The figure shows three views and two pictorial views of one solid part (mm, origin at its lowest corner). Answer the questions. Give positions to 0.01 mm unless a question says otherwise; leave off trailing zeros. Loops run counter-clockwise (first coordinate to the right, second up) from the corner with the lowest first, then second, coordinate; pieces in that order, holes last. Notation, with made-up numbers: M -28,75 L 11,75 A12 ccw 11,90 Z; hole C 86,-24.75 d6. An arc over 180 degrees is marked long. Write item = value, one per line. Start each with the question number.
1. Consider L1, parallel to Y at x = 15, z = 5.5 (3 decimals); L2, parallel to Z at x = 18.5, y = 8.75; L3, parallel to Y at x = 15, z = 17.1. Determine where each line is inside the solid, lowest interval first. Write a range as [from, to].
2. Section D-D on x = 20 is taken. Determine the outline of the cut face in (y, z), plus the area to 3 significant figures.
3. Flat-ended cylindrical pins translate along their axes: pin 1 Ø5 at (x, z) = (26, 12) entering from +Y; pin 2 Ø1 at (x, z) = (18.5, 2.5) entering from -Y; pin 3 Ø3 at (x, y) = (7.5, 5) entering from -Z; pin 4 Ø5 at (y, z) = (16, 11) entering from -X. Find the tip coordinate at first contact, or state that the pin passes through.
4. The mould has two halves that part along Y. Classify the marked faces 1, 2 and 3: released by +Y, released by -Y, zero draft, split by the parting line, or undercut.
5. Section C-C on z = 16.75 is taken. Determine the outline of the cut face in (x, y).
6. Section A-A on x = 15 is taken. Determine the outline of the cut face in (y, z) (3 decimals).
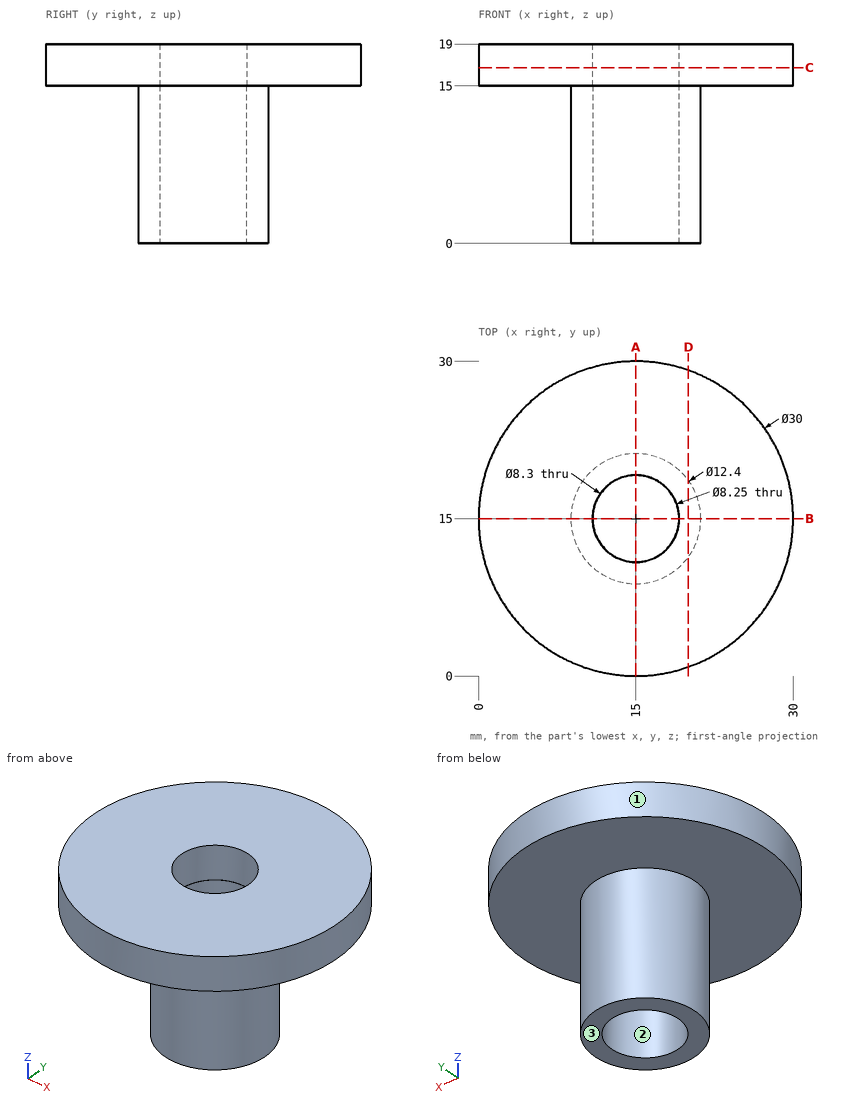
Verdict:
q1.L1 = [8.8, 10.875], [19.125, 21.2]
q1.L2 = [15, 19]
q1.L3 = [0, 10.85], [19.15, 30]
q2.outline = M 0.86,15 L 11.33,15 L 11.33,0 L 18.67,0 L 18.67,15 L 29.14,15 L 29.14,19 L 0.86,19 Z
q2.area = 223 mm2
q3.pin_1 = through
q3.pin_2 = 9.57
q3.pin_3 = 15
q3.pin_4 = 8.8
q4.face_1 = split by the parting line
q4.face_2 = undercut
q4.face_3 = zero draft
q5.outline = C 15,15 d30; hole C 15,15 d8.3
q6.outline = M 0,15 L 8.8,15 L 8.8,0 L 10.875,0 L 10.875,15 L 10.85,15 L 10.85,19 L 0,19 Z; M 19.125,0 L 21.2,0 L 21.2,15 L 30,15 L 30,19 L 19.15,19 L 19.15,15 L 19.125,15 Z
